Input: part model. Units: mm. Frame: model coordinates. A direction names the side the tool comes from. Give positions to 0.01 mm unless a question says otherwise; leave off trailing zeros. Loops run counter-clockwise (first coordinate to the right, second up) from the corner with the lowest first, then second, coordinate; pieces in that order, holes last. Notation, with made-up numbers: (52.25, -39.75) - (108.25, -39.75) arc R14 ccw to (108.25, -30.75) - close; hole circle Ø10 at (48, 25). An arc over 180 degrees is marked (long way). Answer as a JSON object with one key per item and string values. Group by question number.
(1) Section query C-C (y = 0.5). Return loops of the section in (x, z) (3 decimals), plus the area to 3 significant figures.
(2) Material intervals for L1, parallel to X at y = -1, z = -52.5; L2, parallel to Z at x = -33.5, y = 0; L3, parallel to Z at x = -37, y = -1, sorted ascending.
(3) Section query B-B (x = 0). Return loops of the section in (y, z) (3 decimals), plus the area to 3 significant figures.
(4) Access query for faces 1 (the flat face through (2, 3.175, 26)), 2 (the flat face through (0, 0, -50.8)). Directions: +Z, -Z, +X, -X, +Y, -Y. A direction counts if a zero-diameter tool reaches every point of the face in a straight line with its end or side. Return the directions, or none.
(5) Pin query (flat end, axial travel): P1, Ø3, axis at x = 14.5, y = 1, coming from the -Z side. Return the tip coordinate at first contact, or that it passes through.
(6) Section query A-A (z = 0). Return loops of the section in (x, y) (3 decimals), plus the area to 3 significant figures.
(7) Mould query, pull axis Z, two halves, no side actions, for faces 3 (the flat face through (79, 0, -127)), 4 (the flat face through (31.75, 0, -88)), 5 (the cylindrical face through (-11.59, -0.04, -15.12)). Classes: +Z half, -Z half, draft (parallel to the pull), parting line (faces both ways), or undercut.
```python
from build123d import *

# Parameters (mm, degrees)
SKETCH1_R           = 19.05
SKETCH1_R_2         = 6.35
BOSS_EXTRUDE1_DEPTH = 3.175


with BuildPart() as part:
    # Sketch1 → Boss-Extrude1 (new, symmetric)
    with BuildSketch(Plane(origin=(0, 0, 0), x_dir=(1, 0, 0), z_dir=(0, 1, 0))):
        Polygon((-31.75, 50.8), (31.75, 50.8), (31.75, 127), (127, 127), (127, -127), (-127, -127), (-127, 127), (-31.75, 127), align=None)
        with Locations(Location((0, 0, 0), (0, 0, 270))):
            Circle(SKETCH1_R, mode=Mode.SUBTRACT)
        with Locations(Location((-34.925, 34.925, 0), (0, 0, 270))):
            Circle(SKETCH1_R_2, mode=Mode.SUBTRACT)
        with Locations(Location((34.925, 34.925, 0), (0, 0, 90))):
            Circle(SKETCH1_R_2, mode=Mode.SUBTRACT)
        with Locations(Location((34.925, -34.925, 0), (0, 0, 270))):
            Circle(SKETCH1_R_2, mode=Mode.SUBTRACT)
        with Locations(Location((-34.925, -34.925, 0), (0, 0, 90))):
            Circle(SKETCH1_R_2, mode=Mode.SUBTRACT)
    extrude(amount=BOSS_EXTRUDE1_DEPTH, both=True)


solid = part.part
```
Recorded:
{
 "1": {"outline": "(-127, -127) - (-31.75, -127) - (-31.75, -50.8) - (31.75, -50.8) - (31.75, -127) - (127, -127) - (127, 127) - (-127, 127) - close; hole circle Ø12.7 at (-34.925, -34.925); hole circle Ø12.7 at (-34.925, 34.925); hole circle Ø38.1 at (0, 0); hole circle Ø12.7 at (34.925, -34.925); hole circle Ø12.7 at (34.925, 34.925)", "area": "58,000 mm^2"},
 "2": {"L1": "x = -127 to -31.75, 31.75 to 127", "L2": "z = -127 to -41.11, -28.74 to 28.74, 41.11 to 127", "L3": "z = -127 to -40.93, -28.92 to 28.92, 40.93 to 127"},
 "3": {"outline": "(-3.175, -50.8) - (3.175, -50.8) - (3.175, -19.05) - (-3.175, -19.05) - close; (-3.175, 19.05) - (3.175, 19.05) - (3.175, 127) - (-3.175, 127) - close", "area": "887 mm^2"},
 "4": {"face 1": "+Z, -Z, +X, -X, +Y", "face 2": "-Z, +Y, -Y"},
 "5": {"P1": "stops at z = -50.8"},
 "6": {"outline": "(-127, -3.175) - (-19.05, -3.175) - (-19.05, 3.175) - (-127, 3.175) - close; (19.05, -3.175) - (127, -3.175) - (127, 3.175) - (19.05, 3.175) - close", "area": "1,370 mm^2"},
 "7": {"face 3": "-Z half", "face 4": "draft", "face 5": "undercut"}
}
